Source: CAD feature listing. Evaluate the final solid. Frame: model axes, mm. A direction names the side the tool comes from. Round coordinates to 2 decimals unless told otherwise and drop trailing zeros. Order: outer loops, then holes, each group sorted by start corner. A loop starts at its lowest first (then second) coordinate and runs counter-clockwise, first axis right, second up. Notation, with made-up numbers: M -15,-23.75 L -1,-23.75 A23 ccw -1,12.25 Z; hole C 13.5,53.25 d1. An arc over 180 degrees is marked long. Use one line per item in the form item = value. Start each with the question number.
Q1. Pull-direction query (Y, two-part tool) for faces 1 (the flat face through (34.39, -11.76, 12.32)), 2 (the flat face through (-103.65, -39.9, 12.32)), 3 (the flat face through (-53, -5, 0)); classes: pulls with the +Y half, pulls with the -Y half, needs draft (parallel to the pull), parting line crosses it, or undercut.
Q2. Reachability of faces 4 (the flat face through (0.379, -39.353, 12.325)), 5 (the flat face through (-135.924, -11.424, 12.325)), 6 (the flat face through (33.733, 29.826, 12.325)), 7 (the cylindrical face through (47.819, -36.838, 12.325)), 8 (the flat face through (-102.57, 57.755, 12.325)) from +Z, -Z, +X, -X, +Y, -Y: full face, straight path, thin tool, end or side. Return the list, or none.
Q3. Contact query for flat-ended pins moving along their axis: pin 1 (5 mm diameter, centred on x = 0, z = 11, fed in from +Y); pin 2 (1 mm diameter, centred on x = -114, z = 19, fed in from +Y); pin 3 (10 mm diameter, centred on x = 30.5, z = 4.5, fed in from -Y). Output: stop coordinate, or through.
Q4. Section D-D (x = -98.5). Return the cut outline in (y, z), plus the area to 3 significant figures.
Q5. Section A-A (y = 52). Return the cut outline in (x, z), plus the area to 3 significant figures.
Q6. Section C-C (z = 14.5). Return the cut outline in (x, y) (3 decimals).
Q7. Material intervals for probe 1 along X at (y, z) = (62, 22.5); probe 2 along X at (y, z) = (58, 18); probe 3 along Y at (x, z) = (17, 11.5), sorted ascending.
Q8. Section B-B (x = 27). Return the cut outline in (y, z), plus the area to 3 significant figures.
from build123d import *

# Parameters (mm, degrees)
F0_R     = 4.5
F1_DEPTH = 25


with BuildPart() as f1:
    # F0 (on Top) → F1 (new body)
    with BuildSketch(Plane.XY):
        with BuildLine():
            ThreePointArc((48.404608, 55.200653), (51.586588, 56.518673), (52.904608, 59.700653))
            ThreePointArc((52.904608, 59.700653), (45.222627, 62.882634), (48.404608, 55.200653))
        make_face()
        with BuildLine():
            Line((-112.855788, 0.283429), (-159.647047, -23.464898))
            ThreePointArc((-159.647047, -23.464898), (-168.42984, -50.351002), (-141.543737, -59.133795))
            Line((-141.543737, -59.133795), (-64.672874, -20.118935))
            ThreePointArc((-64.672874, -20.118935), (-51.095392, -16.870607), (-37.51791, -20.118935))
            Line((-37.51791, -20.118935), (39.352953, -59.133795))
            ThreePointArc((39.352953, -59.133795), (66.239056, -50.351002), (57.456263, -23.464898))
            Line((57.456263, -23.464898), (10.665003, 0.283429))
            ThreePointArc((10.665003, 0.283429), (5.190831, 9.200653), (10.665003, 18.117877))
            Line((10.665003, 18.117877), (57.456263, 41.866205))
            ThreePointArc((57.456263, 41.866205), (66.239056, 68.752308), (39.352953, 77.535102))
            Line((39.352953, 77.535102), (-37.51791, 38.520241))
            ThreePointArc((-37.51791, 38.520241), (-51.095392, 35.271914), (-64.672874, 38.520241))
            Line((-64.672874, 38.520241), (-141.543737, 77.535102))
            ThreePointArc((-141.543737, 77.535102), (-168.42984, 68.752308), (-159.647047, 41.866205))
            Line((-159.647047, 41.866205), (-112.855788, 18.117877))
            ThreePointArc((-112.855788, 18.117877), (-107.381615, 9.200653), (-112.855788, 0.283429))
        make_face()
        with Locations((-150.595392, -41.299347)):
            Circle(F0_R, mode=Mode.SUBTRACT)
        with Locations((48.404608, -41.299347)):
            Circle(F0_R, mode=Mode.SUBTRACT)
        with Locations((-51.095392, 9.200653)):
            Circle(F0_R, mode=Mode.SUBTRACT)
        with Locations((-150.595392, 59.700653)):
            Circle(F0_R, mode=Mode.SUBTRACT)
        with BuildLine():
            ThreePointArc((48.404608, 55.200653), (45.222627, 62.882634), (52.904608, 59.700653))
            ThreePointArc((52.904608, 59.700653), (51.586588, 56.518673), (48.404608, 55.200653))
        make_face(mode=Mode.SUBTRACT)
    extrude(amount=F1_DEPTH)


solid = f1.part
Results list:
q1.face_1 = undercut
q1.face_2 = pulls with the -Y half
q1.face_3 = needs draft
q2.face_4 = +Z, -Z, -Y
q2.face_5 = +Z, -Z, -X
q2.face_6 = +Z, -Z, +X
q2.face_7 = +Z, -Z
q2.face_8 = +Z, -Z, +Y
q3.pin_1 = 58.83
q3.pin_2 = 63.81
q3.pin_3 = -57.18
q4.outline = M -37.29,0 L 55.69,0 L 55.69,25 L -37.29,25 Z
q4.area = 2,320 mm2
q5.outline = M -169.05,0 L -91.23,0 L -91.23,25 L -169.05,25 Z; M -10.96,0 L 66.86,0 L 66.86,25 L -10.96,25 Z
q5.area = 3,890 mm2
q6.outline = M -159.647,-23.465 A20 ccw -141.544,-59.134 L -64.673,-20.119 A30 cw -37.518,-20.119 L 39.353,-59.134 A20 ccw 57.456,-23.465 L 10.665,0.283 A10 cw 10.665,18.118 L 57.456,41.866 A20 ccw 39.353,77.535 L -37.518,38.52 A30 cw -64.673,38.52 L -141.544,77.535 A20 ccw -159.647,41.866 L -112.856,18.118 A10 cw -112.856,0.283 Z; hole C -150.595,-41.299 d9; hole C -150.595,59.701 d9; hole C -51.095,9.201 d9; hole C 48.405,-41.299 d9; hole M 48.405,55.201 A4.5 ccw 52.905,59.701 A4.5 ccw long Z
q7.probe_1 = -170.46 to -154.46, -146.73 to -110.93, 8.74 to 44.54, 52.27 to 68.27
q7.probe_2 = -170.52 to -154.76, -146.43 to -103.05, 0.86 to 44.24, 52.57 to 68.33
q7.probe_3 = -47.79 to -2.93, 21.33 to 66.19
q8.outline = M -52.86,0 L -8.01,0 L -8.01,25 L -52.86,25 Z; M 26.41,0 L 71.27,0 L 71.27,25 L 26.41,25 Z
q8.area = 2,240 mm2
